CAD build for the part. Positions are in the model's coordinates, mm. Round coordinates to 2 decimals unless told otherwise and drop trailing zeros. Write each loop counter-clockwise with the first axis right and the second up, starting at its lowest first coordinate (ties: lowest second). Pieces come first, ordered by that corner, then holes. Notation, with made-up numbers: M -7.5,-25 L 1.5,-25 A24 ccw 1.5,12 Z; hole C -29.75,79.25 d3. An arc over 180 degrees is marked long. Write each question's results on one line, items separated by ' | '. Start each with the question number.
```python
from build123d import *

# Parameters (mm, degrees)
SKETCH1_R           = 2.35
SKETCH1_R_2         = 5.5
SKETCH1_R_3         = 3.6
SKETCH1_R_4         = 3.8
SKETCH1_W           = 55
SKETCH1_H           = 31
BOSS_EXTRUDE1_DEPTH = 3


with BuildPart() as part:
    # Sketch1 → Boss-Extrude1 (new body)
    with BuildSketch(Plane.XY):
        with BuildLine():
            Line((-95.217720642, 42.05), (-95.217720642, 0))
            Line((-95.217720642, 0), (-111.532377856, -28.257815203))
            ThreePointArc((-111.532377856, -28.257815203), (-117.891374344, -30.093609063), (-120.65, -36.11))
            Line((-120.65, -36.11), (-120.65, -42.05))
            Line((-120.65, -42.05), (-118.65, -44.05))
            Line((-118.65, -44.05), (93.217720642, -44.05))
            Line((93.217720642, -44.05), (95.217720642, -42.05))
            Line((95.217720642, -42.05), (95.217720642, 0))
            Line((95.217720642, 0), (111.532377856, 28.257815203))
            ThreePointArc((111.532377856, 28.257815203), (117.891374344, 30.093609063), (120.65, 36.11))
            Line((120.65, 36.11), (120.65, 42.05))
            Line((120.65, 42.05), (118.65, 44.05))
            Line((118.65, 44.05), (-93.217720642, 44.05))
            Line((-93.217720642, 44.05), (-95.217720642, 42.05))
        make_face()
        with Locations((-112.71, -36.11)):
            Circle(SKETCH1_R, mode=Mode.SUBTRACT)
        with Locations((-80.357720642, -22.025)):
            Circle(SKETCH1_R_2, mode=Mode.SUBTRACT)
        with Locations((-37.5, -33.344646258)):
            Circle(SKETCH1_R_3, mode=Mode.SUBTRACT)
        with BuildLine():
            ThreePointArc((-30.35, -32.594646258), (-29.7, -31.944646258), (-29.05, -32.594646258))
            Line((-29.05, -32.594646258), (-29.05, -34.094646258))
            ThreePointArc((-29.05, -34.094646258), (-29.7, -34.744646258), (-30.35, -34.094646258))
            Line((-30.35, -34.094646258), (-30.35, -32.594646258))
        make_face(mode=Mode.SUBTRACT)
        with Locations((-12.5, -33.344646258)):
            Circle(SKETCH1_R_3, mode=Mode.SUBTRACT)
        with BuildLine():
            Line((-5.35, -34.094646258), (-5.35, -32.594646258))
            ThreePointArc((-5.35, -32.594646258), (-4.7, -31.944646258), (-4.05, -32.594646258))
            Line((-4.05, -32.594646258), (-4.05, -34.094646258))
            ThreePointArc((-4.05, -34.094646258), (-4.7, -34.744646258), (-5.35, -34.094646258))
        make_face(mode=Mode.SUBTRACT)
        with Locations((12.5, -33.344646258)):
            Circle(SKETCH1_R_3, mode=Mode.SUBTRACT)
        with BuildLine():
            Line((19.65, -34.094646258), (19.65, -32.594646258))
            ThreePointArc((19.65, -32.594646258), (20.3, -31.944646258), (20.95, -32.594646258))
            Line((20.95, -32.594646258), (20.95, -34.094646258))
            ThreePointArc((20.95, -34.094646258), (20.3, -34.744646258), (19.65, -34.094646258))
        make_face(mode=Mode.SUBTRACT)
        with Locations((37.5, -33.344646258)):
            Circle(SKETCH1_R_3, mode=Mode.SUBTRACT)
        with BuildLine():
            Line((44.65, -34.094646258), (44.65, -32.594646258))
            ThreePointArc((44.65, -32.594646258), (45.3, -31.944646258), (45.95, -32.594646258))
            Line((45.95, -32.594646258), (45.95, -34.094646258))
            ThreePointArc((45.95, -34.094646258), (45.3, -34.744646258), (44.65, -34.094646258))
        make_face(mode=Mode.SUBTRACT)
        with Locations((80.358860321, -22.025)):
            Circle(SKETCH1_R_2, mode=Mode.SUBTRACT)
        with Locations((-80.357720642, 0)):
            Circle(SKETCH1_R_2, mode=Mode.SUBTRACT)
        with Locations((40.137585267, 5.460707483)):
            Circle(SKETCH1_R_4, mode=Mode.SUBTRACT)
        with Locations((0, 10.05)):
            Rectangle(SKETCH1_W, SKETCH1_H, mode=Mode.SUBTRACT)
        with BuildLine():
            ThreePointArc((74.858860321, 0), (80.358860321, 5.5), (85.858860321, 0))
            ThreePointArc((85.858860321, 0), (80.358860321, -5.5), (74.858860321, 0))
        make_face(mode=Mode.SUBTRACT)
        with Locations((112.71, 36.11)):
            Circle(SKETCH1_R, mode=Mode.SUBTRACT)
        with BuildLine():
            ThreePointArc((-54.993253468, -16.61863742), (-55.643253468, -17.26863742), (-56.293253468, -16.61863742))
            Line((-56.293253468, -16.61863742), (-56.293253468, -15.11863742))
            ThreePointArc((-56.293253468, -15.11863742), (-55.643253468, -14.46863742), (-54.993253468, -15.11863742))
            Line((-54.993253468, -15.11863742), (-54.993253468, -16.61863742))
        make_face(mode=Mode.SUBTRACT)
        with Locations((-63.443253468, -15.86863742)):
            Circle(SKETCH1_R_3, mode=Mode.SUBTRACT)
    extrude(amount=BOSS_EXTRUDE1_DEPTH)


solid = part.part
```
1) Wall check: line 1 along Y through (x, z) = (12.5, 1.45); line 2 along X through (y, z) = (-1.5, 2); line 3 along Y through (x, z) = (-37.5, 1.05). Give the ranges that are in metal, low to high. Write a range as from..to.
2) Saw through at B-B, the plane x = 82. Write the cut outline in (y, z), plus the area to 3 significant figures.
3) Saw through at D-D, the plane z = 1.5. State how many separate pieces and enclosed holes the cut face has, plus the area to 3 significant figures.
4) Drop flat-ended pins along their axis: pin 1 Ø0.8 at (y, z) = (-33.5, 2) entering from -X; pin 2 Ø1.5 at (y, z) = (13.5, 1.5) entering from -X; pin 3 Ø0.8 at (y, z) = (-33, 1) entering from -X. Give the stop position or say it passes through.
5) Saw through at C-C, the plane x = 2. Write the cut outline in (y, z), plus the area to 3 significant figures.
6) Pull direction X, two halves, no side cores. Call faces 1 (the face through (-2, -9, 0)), 2 (the face through (-37.969, -29.775, 1.479)): pulls with the +X half, pulls with the -X half, needs draft (parallel to the pull), parting line crosses it, or undercut.
7) Saw through at A-A, the plane x = -37.5. Write the cut outline in (y, z), plus the area to 3 significant figures.
Filled sheet:
1) line 1: y = -44.05..-36.94, -29.74..-5.45, 25.55..44.05 | line 2: x = -96.08..-85.65, -75.07..-27.5, 27.5..75.07, 85.65..95.22 | line 3: y = -44.05..-36.94, -29.74..44.05
2) outline: M -44.05,0 L -27.27,0 L -27.27,3 L -44.05,3 Z; M -16.78,0 L -5.25,0 L -5.25,3 L -16.78,3 Z; M 5.25,0 L 44.05,0 L 44.05,3 L 5.25,3 Z | area: 201 mm^2
3) separate pieces: 1 | enclosed holes: 18 | area: 15,600 mm^2
4) pin 1: stops at x = -120.34 | pin 2: stops at x = -95.22 | pin 3: stops at x = -120.17
5) outline: M -44.05,0 L -5.45,0 L -5.45,3 L -44.05,3 Z; M 25.55,0 L 44.05,0 L 44.05,3 L 25.55,3 Z | area: 171 mm^2
6) face 1: needs draft | face 2: undercut
7) outline: M -44.05,0 L -36.94,0 L -36.94,3 L -44.05,3 Z; M -29.74,0 L 44.05,0 L 44.05,3 L -29.74,3 Z | area: 243 mm^2
